Here's how the part is built. I have some questions about the finished solid (model axes, mm). A direction names the side the tool comes from. Round coordinates to 2 decimals unless told otherwise and drop trailing zeros. Write each loop counter-clockwise with the first axis right and the second up, starting at its lowest first coordinate (ties: lowest second). Pieces come first, ordered by that corner, then holes. Notation, with made-up numbers: (51.25, -34) - (68.25, -34) arc R16 ccw to (68.25, -5) - close; hole circle Ø3 at (23.5, 48.5). An arc over 180 degrees is marked (long way). Write item = value, one per line. Start each with the question number.
Item 1: If I drill on line 1 along X through (y, z) = (-13.75, 1.75); line 2 along X through (y, z) = (-2.75, 7.25); line 3 along X through (y, z) = (-13.5, 9.5), over which ranges is the centre line in solid material (lowest first)? Write a range as [from, to].
Item 2: If we section it at A-A (x = -49.5): Please give me the cut outline in (y, z), and give its area (3 significant figures).
Item 3: Which directions (+Z, -Z, +X, -X, +Y, -Y) give clear straight access to the entire face, cutting with the end or side of a thin tool? Please do faces 5 (the face through (-35, -17, 2)), 6 (the face through (-59.058, -9, 5)), 7 (the face through (50, -13.734, 7)), 8 (the face through (-2, -12, 0)), 9 (the face through (-45, -10.734, 5)).
Item 4: For P1, Ø7, axis at x = 30.94, y = -16.78, coming from the +Z side; P2, Ø2.5, axis at x = -54, z = 6.5, coming from the +Y side, each with a flat end and sliding along its axis, tell me the tip position at first contact or that it passes through.
Item 5: Thinking about a two-plate mould opening in X: for faces 1 (the face through (-57.63, -20.23, 5.07)), 2 (the face through (-46.558, -15, 5)), 3 (the face through (-48.558, -15, 5)), 4 (the face through (55.942, -9, 5)), which applies, pulls with the +X half, pulls with the -X half, needs draft (parallel to the pull), parting line crosses it, or undercut?
Item 6: If we section it at B-B (z = 3): Please give me the cut outline in (x, y).
```python
from build123d import *

# Parameters (mm, degrees)
F0_W     = 115
F0_H     = 20
F1_DEPTH = 10
F2_R     = 4
F3_DEPTH = 8
F4_R     = 1.5
F5_DEPTH = 12
F6_R     = 5
F7_W     = 2.5
F7_H     = 8
F8_DEPTH = 25
F9_R     = 0.99999


# Not quite as in the source:
# - a fillet or chamfer is up to 0.001 mm smaller than in the source, because OpenCascade refuses the exact size


with BuildPart() as f1:
    # F0 (on Top) → F1 (new body)
    with BuildSketch(Plane.XY):
        with Locations((-1.558380723, -11.7337754572)):
            Rectangle(F0_W, F0_H)
    extrude(amount=F1_DEPTH)

    # F2 (on face) → F3 (cut)
    with BuildSketch(Plane.XY.offset(10)):
        with Locations((-35.058380723, -16.7792532593)):
            Circle(F2_R)
        with Locations((30.941619277, -16.7792532593)):
            Circle(F2_R)
    extrude(amount=-F3_DEPTH, mode=Mode.SUBTRACT)

    # F4 (on face) → F5 (cut)
    with BuildSketch(Plane(origin=(0, -1.7337754572, 0), x_dir=(-1, 0, 0), z_dir=(0, 1, 0))):
        with Locations((54.058380723, 6.6987262902)):
            Circle(F4_R)
        with Locations((-49.941619277, 6.6987262902)):
            Circle(F4_R)
    extrude(amount=-F5_DEPTH, mode=Mode.SUBTRACT)

    # F6
    f6_edges = [f1.edges().sort_by_distance(p)[0] for p in [
        (-59.058381, -21.733775, 5),
        (55.941619, -21.733775, 5),
    ]]
    fillet(f6_edges, radius=F6_R)

    # F7 (on face) → F8 (cut)
    with BuildSketch(Plane.XY.offset(10)):
        with Locations((-49.808380723, -14.7337754572)):
            Rectangle(F7_W, F7_H)
        with Locations((-45.308380723, -14.7337754572)):
            Rectangle(F7_W, F7_H)
    extrude(amount=-F8_DEPTH, mode=Mode.SUBTRACT)

    # F9 (radius 1 in the source; OpenCascade refuses exactly that, so slightly less here)
    f9_edges = [f1.edges().sort_by_distance(p)[0] for p in [
        (-51.058381, -14.733775, 10),
        (-49.808381, -10.733775, 10),
        (-48.558381, -14.733775, 10),
        (-49.808381, -18.733775, 10),
        (-45.308381, -18.733775, 10),
        (-46.558381, -14.733775, 10),
        (-45.308381, -10.733775, 10),
        (-44.058381, -14.733775, 10),
        (-44.058381, -14.733775, 0),
        (-45.308381, -10.733775, 0),
        (-46.558381, -14.733775, 0),
        (-45.308381, -18.733775, 0),
        (-49.808381, -18.733775, 0),
        (-48.558381, -14.733775, 0),
        (-49.808381, -10.733775, 0),
        (-51.058381, -14.733775, 0),
    ]]
    fillet(f9_edges, radius=F9_R)


solid = f1.part
```
Reply:
q1.line_1 = [-59.06, -51.06], [-48.56, -46.56], [-44.06, 55.94]
q1.line_2 = [-59.06, -55.45], [-52.66, 48.55], [51.34, 55.94]
q1.line_3 = [-59.06, -51.19], [-48.42, -46.69], [-43.92, -37.35], [-32.77, 28.65], [33.23, 55.94]
q2.outline = (-21.73, 0) - (-19.73, 0) arc R1 ccw to (-18.73, 1) - (-18.73, 9) arc R1 ccw to (-19.73, 10) - (-21.73, 10) - close; (-10.73, 1) arc R1 ccw to (-9.73, 0) - (-1.73, 0) - (-1.73, 10) - (-9.73, 10) arc R1 ccw to (-10.73, 9) - close
q2.area = 119 mm2
q3.face_5 = +Z
q3.face_6 = +Z, -Z, -X, +Y, -Y
q3.face_7 = +Y
q3.face_8 = -Z, +X, -X, +Y, -Y
q3.face_9 = +Z, -Z
q4.P1 = 2
q4.P2 = -13.73
q5.face_1 = pulls with the -X half
q5.face_2 = undercut
q5.face_3 = undercut
q5.face_4 = pulls with the +X half
q6.outline = (-59.06, -16.73) arc R5 ccw to (-54.06, -21.73) - (50.94, -21.73) arc R5 ccw to (55.94, -16.73) - (55.94, -1.73) - (-59.06, -1.73) - close; hole (-51.06, -18.73) - (-48.56, -18.73) - (-48.56, -10.73) - (-51.06, -10.73) - close; hole (-46.56, -18.73) - (-44.06, -18.73) - (-44.06, -10.73) - (-46.56, -10.73) - close; hole circle Ø8 at (-35.06, -16.78); hole circle Ø8 at (30.94, -16.78)
